The listing builds one solid part. Answer for the finished solid, in the listing's coordinates (mm). Face numbers are marked on the shaded views. A direction names the side the tool comes from. Give positions to 0.01 mm unless a question says otherwise; leave off trailing zeros. Loops run counter-clockwise (first coordinate to the right, second up) from the corner with the lowest first, then second, coordinate; pieces in that order, holes last.
Item 1: Section D-D, the plane x = 23 is taken. Give the vertices of the cut face in (y, z).
Item 2: Section B-B, the plane z = -49 is taken. Give the vertices of the cut face in (x, y), and give its area (3 significant figures).
Item 3: Each of these flat-tipped pins is pushed along its axis until it touches: pin 1 Ø6.5 at (x, z) = (0, 0) entering from +Y; pin 2 Ø5 at (x, z) = (19.5, -18) entering from +Y; pin 3 Ø1.5 at (x, z) = (98.5, 0) entering from +Y; pin 4 Ø4 at (x, y) = (9.02, 36.59) entering from +Z. Where does it stop, or does it pass through?
Item 4: Consider line 1 along X through (y, z) = (21.5, -90); line 2 along X through (y, z) = (36.5, -39); line 3 along Z through (x, y) = (19, 16.5). Determine where each line is inside the solid, lowest interval first.
Item 5: A tool of negligible diameter and unlimited length cuts with its end or side. For the marked faces 4 and 5, from which of +Z, -Z, +X, -X, +Y, -Y can it reach the whole face along a straight path? Write none if from no direction.
Item 6: Section A-A, the plane x = 65 is taken. Give the vertices of the cut face in (y, z).
Item 7: Section C-C, the plane y = 27 is taken. Give the vertices of the cut face in (x, z).
Item 8: The mould has two halves that part along Z. Classify the marked faces 1, 2 and 3: pulls with the +Z half, pulls with the -Z half, needs draft (parallel to the pull), parting line crosses it, or undercut.
Autodesk Inventor part; units mm, degrees
ref_plane "YZ Plane" through (0, 0, 0) normal (1, 0, 0) x (0, 1, 0)
ref_plane "XZ Plane" through (0, 0, 0) normal (0, 1, 0) x (-1, 0, 0)
ref_plane "XY Plane" through (0, 0, 0) normal (0, 0, 1) x (1, 0, 0)
sketch "Sketch1" plane through (0, 0, 0) normal (0, 1, 0) x (-1, 0, 0)
  line L0 (0, 0) -> (-98, 0)
  line L1 (-98, 0) -> (-98, -100)
  line L2 (-98, -100) -> (0, -100)
  line L3 (0, -100) -> (0, 0)
  line L4 (3, -103) -> (-101, -103)
  line L5 (-101, -103) -> (-101, 3)
  line L6 (-101, 3) -> (3, 3)
  line L7 (3, 3) -> (3, -103)
  line L8 (0, -20) -> (-6, -20)
  line L9 (-6, -20) -> (-6, -80)
  line L10 (-6, -80) -> (0, -80)
  line L11 (0, -80) -> (0, -20)
  line L12 (-46, -20) -> (-52, -20)
  line L13 (-52, -20) -> (-52, -80)
  line L14 (-52, -80) -> (-46, -80)
  line L15 (-46, -80) -> (-46, -20)
  line L16 (-92, -20) -> (-98, -20)
  line L17 (-98, -20) -> (-98, -80)
  line L18 (-98, -80) -> (-92, -80)
  line L19 (-92, -80) -> (-92, -20)
  point P0 (-49, -20)
  point P1 (-6, -50)
  point P2 (-98, -20)
  point P3 (-98, -80)
  point P4 (0, -80)
  point P5 (0, -20)
  dimension "d0" = 100
  dimension "d1" = 98
  dimension "d2" = 3
  dimension "d48" = 6
  dimension "d49" = 60
  dimension "d50" = 6
  dimension "d51" = 60
  dimension "d52" = 6
  dimension "d53" = 60
  dimension "d54" = 49
  dimension "d55" = 50
extrude "Extrusion1" add sketch "Sketch1" along normal blind 4 contours L3 L8 L9 L10 L2 L1 L18 L19 L16 L0 | L3 L10 L9 L8 | L16 L19 L18 L1 | L15 L14 L13 L12
extrude "Extrusion2" add sketch "Sketch1" along normal blind 55 contours L4 L5 L6 L7
fillet "Fillet1" radius 2 4 edges at (-3, 27.5, 3) (101, 27.5, 3) (101, 27.5, -103) (-3, 27.5, -103)
sketch "Sketch2" plane through (0, 4, 0) normal (0, 1, 0) x (1, 0, 0)
  line L0 (98, 0) -> (98, 100)
  line L1 (98, 100) -> (0, 100)
  line L2 (0, 100) -> (0, 0)
  line L3 (0, 0) -> (98, 0)
  circle A0 centre (5.185, 73.913) radius 3
  circle A1 centre (5.185, 6.858) radius 3
  circle A2 centre (92.815, 6.858) radius 3
  circle A3 centre (92.815, 73.913) radius 3
  line L4 (54.5, 100) -> (51.5, 100)
  line L5 (51.5, 100) -> (51.5, 85)
  line L6 (51.5, 85) -> (54.5, 85)
  line L7 (54.5, 85) -> (54.5, 100)
  line L8 (0, 100) -> (98, 100)
  dimension "d8" = 6
  dimension "d9" = 6
  dimension "d10" = 6
  dimension "d11" = 6
  dimension "d12" = 67.055
  dimension "d13" = 87.63
  dimension "d16" = 6.858
  dimension "d17" = 5.185
  dimension "d120" = 3
  dimension "d121" = 15
  dimension "d122" = 51.5
extrude "Extrusion3" add sketch "Sketch2" along normal blind 19 contours L7 L6 L5 L1 | A0 | A1 | A2 | A3
sketch "Sketch3" plane through (92.815, 23, -73.913) normal (0, 1, 0) x (1, 0, 0)
  circle A0 centre (0, -67.055) radius 3
  circle A1 centre (0, -67.055) radius 1.05
  circle A2 centre (0, 0) radius 3
  circle A3 centre (0, 0) radius 1.05
  circle A4 centre (-87.63, 0) radius 3
  circle A5 centre (-87.63, 0) radius 1.05
  circle A6 centre (-87.63, -67.055) radius 3
  circle A7 centre (-87.63, -67.055) radius 1.05
  point P0 (-92.815, -73.913)
  dimension "d21" = 2.1
  dimension "d22" = 2.1
  dimension "d23" = 2.1
  dimension "d24" = 2.1
extrude "Extrusion4" cut sketch "Sketch3" against normal blind 5 contours A1 | A3 | A5 | A7
fillet "Fillet2" radius 2 4 edges at (89.815, 4, -73.913) (89.815, 4, -6.858) (2.185, 4, -6.858) (2.185, 4, -73.913)
extrude "Extrusion5" cut sketch "Sketch1" along normal blind 2 contours L3 L10 L9 L8 | L16 L19 L18 L1 | L15 L14 L13 L12
sketch "Sketch4" plane through (-1, 0, 3) normal (0, 0, 1) x (1, 0, 0)
  line L0 (11.185, 4) -> (1.185, 4)
  line L1 (98.815, 4) -> (88.815, 4)
  line L2 (99, 4) -> (55.5, 4)
  line L3 (1, 4) -> (99, 4)
  line L4 (98.815, 4) -> (88.815, 4)
  line L5 (11.185, 4) -> (1.185, 4)
  line L6 (1, 4) -> (1, 55)
  line L7 (1, 4) -> (1, 55)
  line L8 (99, 4) -> (99, 55)
  line L9 (99, 4) -> (99, 55)
  line L10 (45.1, 47) -> (33, 47)
  line L11 (33, 47) -> (33, 36)
  line L12 (33, 36) -> (45.1, 36)
  line L13 (45.1, 36) -> (45.1, 47)
  line L14 (49.315, 6) -> (60.315, 6)
  line L15 (60.315, 6) -> (60.315, 12)
  line L16 (60.315, 12) -> (49.315, 12)
  line L17 (49.315, 12) -> (49.315, 6)
  line L18 (64.5, 47) -> (73.5, 47)
  line L19 (73.5, 47) -> (73.5, 36)
  line L20 (73.5, 36) -> (64.5, 36)
  line L21 (64.5, 36) -> (64.5, 47)
  line L22 (9.185, 23) -> (3.185, 23)
  line L23 (96.815, 23) -> (90.815, 23)
  circle A0 centre (10.0225, 36.5908) radius 2.5
  circle A1 centre (10.0225, 44.8769) radius 2.5
  line L24 (82.6763, 48.8494) -> (94.9263, 48.8494)
  line L25 (94.9263, 48.8494) -> (94.9263, 29.8494)
  line L26 (94.9263, 29.8494) -> (82.6763, 29.8494)
  line L27 (82.6763, 29.8494) -> (82.6763, 48.8494)
  line L28 (82.6763, 48.8494) -> (94.9263, 29.8494) construction
  line L29 (94.9263, 48.8494) -> (82.6763, 29.8494) construction
  line L30 (0, 0) -> (100, 0)
  line L31 (55.5, 4) -> (52.5, 4)
  line L32 (52.5, 4) -> (1, 4)
  point P0 (1, 0)
  point P1 (69, 36)
  point P2 (73.5, 41.5)
  point P3 (60.315, 9)
  point P4 (49.315, 9)
  point P5 (54.815, 6)
  point P6 (54.815, 12)
  point P7 (6.185, 23)
  point P8 (39.05, 36)
  point P9 (93.815, 23)
  point P10 (88.8013, 39.3494)
  dimension "d56" = 11
  dimension "d57" = 19.4
  dimension "d59" = 12.1
  dimension "d60" = 11
  dimension "d61" = 9
  dimension "d62" = 11
  dimension "d63" = 6
  dimension "d106" = 39
  dimension "d108" = 5
  dimension "d109" = 5
  dimension "d111" = 12.25
  dimension "d112" = 19
  dimension "d117" = 32
  dimension "d118" = 47
  dimension "d119" = 12
extrude "Extrusion6" cut sketch "Sketch4" against normal up to surface (3 mm away)
sketch "Sketch5" plane through (101, 0, 1) normal (1, 0, 0) x (0, 0, -1)
  line L0 (12.858, 4) -> (2.858, 4)
  line L1 (79.913, 4) -> (69.913, 4)
  line L2 (1, 4) -> (101, 4)
  line L3 (101, 4) -> (1, 4)
  line L4 (12.858, 4) -> (2.858, 4)
  line L5 (79.913, 4) -> (69.913, 4)
  line L6 (1, 36) -> (1, 47)
  line L7 (1, 47) -> (1, 36)
  line L8 (1, 47) -> (1, 36)
  line L9 (1, 36) -> (1, 47)
  line L10 (1, 4) -> (1, 55)
  line L11 (1, 4) -> (1, 55)
  line L12 (10.858, 23) -> (4.858, 23)
  line L13 (77.913, 23) -> (71.913, 23)
  line L14 (19.133, 24.6) -> (69.133, 24.6)
  line L15 (69.133, 24.6) -> (69.133, 34.6)
  line L16 (69.133, 34.6) -> (19.133, 34.6)
  line L17 (19.133, 34.6) -> (19.133, 24.6)
  line L18 (12.858, 4) -> (2.858, 4)
  line L19 (4.858, 6) -> (10.858, 6)
  line L20 (79.913, 4) -> (69.913, 4)
  line L21 (71.913, 6) -> (77.913, 6)
  line L22 (1, 12) -> (1, 6)
  line L23 (1, 6) -> (1, 12)
  line L24 (101, 4) -> (86, 4)
  line L25 (86, 4) -> (101, 4)
  point P0 (1, 0)
  point P1 (74.913, 23)
  dimension "d1" = 98
  dimension "d98" = 10
  dimension "d99" = 50
  dimension "d101" = 1.6
  dimension "d102" = 5.78
sketch "Sketch6" plane through (-3, 0, -101) normal (-1, 0, 0) x (0, 0, 1)
  line L0 (32.867, 34.6) -> (82.867, 34.6)
  line L1 (32.867, 24.6) -> (32.867, 34.6)
  line L2 (82.867, 24.6) -> (32.867, 24.6)
  line L3 (82.867, 34.6) -> (82.867, 24.6)
  point P0 (101, 0)
extrude "Extrusion7" cut sketch "Sketch5" against normal up to surface (3 mm away)
extrude "Extrusion8" cut sketch "Sketch6" against normal up to surface (3 mm away)
sketch "Sketch7" plane through (0, 55, 0) normal (0, 1, 0) x (1, 0, 0)
  circle A0 centre (0, 100) radius 2.5
  circle A1 centre (0, 0) radius 2.5
  line L0 (98, 100) -> (98, 0)
  circle A2 centre (98, 100) radius 2.5
  circle A3 centre (98, 0) radius 2.5
  dimension "d113" = 5
  dimension "d114" = 5
  dimension "d115" = 5
  dimension "d116" = 5
extrude "Extrusion9" cut sketch "Sketch7" against normal blind 1.5
fillet "Fillet3" radius 2 6 edges at (51.5, 4, -92.5) (53, 4, -85) (54.5, 4, -92.5) (54.5, 13.5, -100) (51.5, 13.5, -100) (53, 23, -100)
properties part number "Base Chassis"
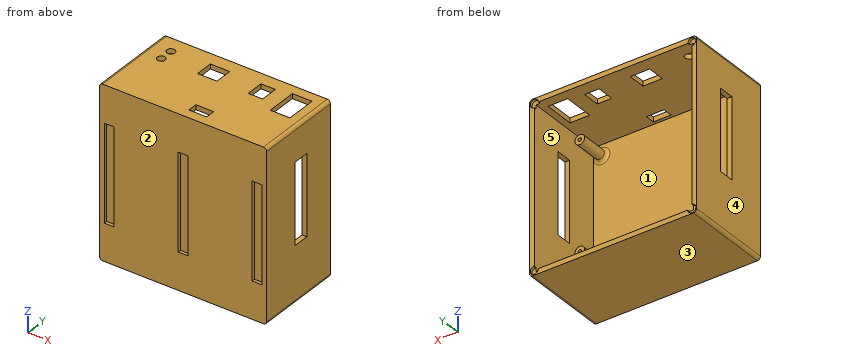
Worked answers:
1. outline: (0, -103) - (55, -103) - (55, -100) - (4, -100) - (4, 0) - (55, 0) - (55, 3) - (0, 3) - close
2. outline: (-3, 0) - (0, 0) - (0, 2) - (6, 2) - (6, 0) - (46, 0) - (46, 2) - (52, 2) - (52, 0) - (92, 0) - (92, 2) - (98, 2) - (98, 0) - (101, 0) - (101, 24.6) - (98, 24.6) - (98, 4) - (0, 4) - (0, 24.6) - (-3, 24.6) - close; (-3, 34.6) - (0, 34.6) - (0, 55) - (-3, 55) - close; (98, 34.6) - (101, 34.6) - (101, 55) - (98, 55) - close
2. area: 626 mm2
3. pin 1: stops at y = 55
3. pin 2: stops at y = 4
3. pin 3: stops at y = 53.5
3. pin 4: stops at z = -100
4. line 1: x = -3 to 0, 51.5 to 54.5, 98 to 101
4. line 2: x = -3 to 0, 98 to 101
4. line 3: z = -103 to -100, 0 to 3
5. face 4: +Z, -Z, -X, +Y, -Y
5. face 5: +Y
6. outline: (0, -103) - (55, -103) - (55, -100) - (4, -100) - (4, 0) - (36, 0) - (36, 3) - (0, 3) - close; (47, 0) - (55, 0) - (55, 3) - (47, 3) - close
7. outline: (-3, -101) arc R2 ccw to (-1, -103) - (99, -103) arc R2 ccw to (101, -101) - (101, -68.13) - (98, -68.13) - (98, -100) - (0, -100) - (0, -68.13) - (-3, -68.13) - close; (-3, -18.13) - (0, -18.13) - (0, 0) - (98, 0) - (98, -18.13) - (101, -18.13) - (101, 1) arc R2 ccw to (99, 3) - (-1, 3) arc R2 ccw to (-3, 1) - close
8. face 1: undercut
8. face 2: needs draft
8. face 3: pulls with the -Z half
